```python
from build123d import *

# Parameters (mm, degrees)
SKETCH2_R          = 1.25
CUT_EXTRUDE1_DEPTH = 21.98
SKETCH3_R          = 2.5
CUT_EXTRUDE2_DEPTH = 15.98
SKETCH4_R          = 9.5
CUT_EXTRUDE3_DEPTH = 10
FILLET1_R          = 2
FILLET2_R          = 2


with BuildPart() as part:
    # Sketch1 → Revolve1 (revolve)
    with BuildSketch(Plane(origin=(0, 0, 0), x_dir=(1, 0, 0), z_dir=(0, 1, 0))):
        Polygon((7.143835403, 5.9), (7.143835403, 13.4), (4.13367975, 18), (-13.836164597, 18), (-13.836164597, 0), (7.143835403, 0), (11.143835403, 0), (11.143835403, 5.9), align=None)
    revolve(axis=Axis((-26.115988439, 0, 0), (1, 0, 0)))

    # Sketch2 → Cut-Extrude1 (cut, through all)
    with BuildSketch(Plane(origin=(7.143835403, 0, 0), x_dir=(0, 0, -1), z_dir=(1, 0, 0))):
        with Locations((0, 11.5)):
            Circle(SKETCH2_R)
        with Locations((8.131727984, 8.131727984)):
            Circle(SKETCH2_R)
        with Locations((11.5, 0)):
            Circle(SKETCH2_R)
        with Locations((8.131727984, -8.131727984)):
            Circle(SKETCH2_R)
        with Locations((0, -11.5)):
            Circle(SKETCH2_R)
        with Locations((-8.131727984, -8.131727984)):
            Circle(SKETCH2_R)
        with Locations((-11.5, 0)):
            Circle(SKETCH2_R)
        with Locations((-8.131727984, 8.131727984)):
            Circle(SKETCH2_R)
    extrude(amount=-CUT_EXTRUDE1_DEPTH, mode=Mode.SUBTRACT)

    # Sketch3 → Cut-Extrude2 (cut)
    with BuildSketch(Plane.ZY.offset(13.836164597)):
        with Locations((0, 11.5)):
            Circle(SKETCH3_R)
        with Locations((8.131727984, 8.131727984)):
            Circle(SKETCH3_R)
        with Locations((11.5, 0)):
            Circle(SKETCH3_R)
        with Locations((8.131727984, -8.131727984)):
            Circle(SKETCH3_R)
        with Locations((0, -11.5)):
            Circle(SKETCH3_R)
        with Locations((-8.131727984, -8.131727984)):
            Circle(SKETCH3_R)
        with Locations((-11.5, 0)):
            Circle(SKETCH3_R)
        with Locations((-8.131727984, 8.131727984)):
            Circle(SKETCH3_R)
    extrude(amount=-CUT_EXTRUDE2_DEPTH, mode=Mode.SUBTRACT)

    # Sketch4 → Cut-Extrude3 (cut)
    with BuildSketch(Plane.ZY.offset(13.836164597)):
        Circle(SKETCH4_R)
    extrude(amount=-CUT_EXTRUDE3_DEPTH, mode=Mode.SUBTRACT)

    # Fillet1
    fillet1_edges = [part.edges().sort_by_distance(p)[0] for p in [
        (11.143835403, 0, 5.9),
    ]]
    fillet(fillet1_edges, radius=FILLET1_R)

    # Fillet2
    fillet2_edges = [part.edges().sort_by_distance(p)[0] for p in [
        (4.13367975, 0, 18),
    ]]
    fillet(fillet2_edges, radius=FILLET2_R)


solid = part.part
```
The model under review builds one solid part; all positions refer to its coordinate system, in mm. A direction names the side the tool comes from. Give positions to 0.01 mm unless a question says otherwise; leave off trailing zeros. Write each loop counter-clockwise with the first axis right and the second up, starting at its lowest first coordinate (ties: lowest second). Pieces come first, ordered by that corner, then holes.
(1) The part is to be moulded in two halves that separate along Y. For faces 1 (the cylindrical face through (-5.958, 10.24, 9.476)), 2 (the flat face through (7.144, 0.2, -6.1)), 3 (the conical face through (6.993, 4.094, -13.002)), say which applies: released by +Y, released by -Y, zero draft, split by the parting line, or undercut.
(2) Tool access review of faces 4 (the cylindrical face through (4.68, 6.91, 8.4)), 5 (the cylindrical face through (-5.958, 0.751, 13.885)): name each direction out of +Z, -Z, +X, -X, +Y, -Y from which nothing blocks a thin tool from reaching the whole face with its end or side.
(3) For P1, Ø2, axis at y = 13.5, z = -2, coming from the +X side; P2, Ø1.5, axis at y = 0.5, z = -12.5, coming from the -X side; P3, Ø2, axis at y = 11.5, z = 0, coming from the +X side; P4, Ø5, axis at x = 1, y = -12, coming from the +Z side, all flat-tipped, find the tip position at first contact; note any pin that passes through.
(4) Consider section A-A, the plane x = -8.75. Give the boundary of the cut face in (y, z), and give its area (3 significant figures).
(5) Consider section B-B, the plane y = 0. Give the number of separate pieces and of enclosed holes in the cut face, and give its area (3 significant figures).
(6) To check wall thickness, follow L1, parallel to Z at x = -2.5, y = 0; L2, parallel to Z at x = -2, y = 6; L3, parallel to Y at x = 4.75, z = 0. State the ranges of each line that lie inside material, in increasing order.
Returned:
1. face 1: undercut
1. face 2: zero draft
1. face 3: split by the parting line
2. face 4: +X, -X
2. face 5: -X
3. P1: stops at x = 7.14
3. P2: stops at x = 2.14
3. P3: passes through
3. P4: stops at z = 15.29
4. outline: circle Ø36 at (0, 0); hole (-9.4, -1.36) arc R9.5 ccw to (-7.61, -5.69) arc R2.5 ccw (long way) to (-5.69, -7.61) arc R9.5 ccw to (-1.36, -9.4) arc R2.5 ccw (long way) to (1.36, -9.4) arc R9.5 ccw to (5.69, -7.61) arc R2.5 ccw (long way) to (7.61, -5.69) arc R9.5 ccw to (9.4, -1.36) arc R2.5 ccw (long way) to (9.4, 1.36) arc R9.5 ccw to (7.61, 5.69) arc R2.5 ccw (long way) to (5.69, 7.61) arc R9.5 ccw to (1.36, 9.4) arc R2.5 ccw (long way) to (-1.36, 9.4) arc R9.5 ccw to (-5.69, 7.61) arc R2.5 ccw (long way) to (-7.61, 5.69) arc R9.5 ccw to (-9.4, 1.36) arc R2.5 ccw (long way) to start
4. area: 585 mm2
5. separate pieces: 3
5. enclosed holes: 0
5. area: 422 mm2
6. L1: z = -18 to -14, -9 to 9, 14 to 18
6. L2: z = -16.97 to -9.44, -6.83 to 6.83, 9.44 to 16.97
6. L3: y = -17.06 to -12.75, -10.25 to 10.25, 12.75 to 17.06
